Here's the drawing with two shaded views (mm, measured from the low corner). I have some questions. A direction names the side the tool comes from. Coordinates: 2 decimals unless noted, no trailing zeros. Order: outer loops, then holes, each group sorted by start corner. A loop starts at its lowest first (then second) coordinate and runs counter-clockwise, first axis right, second up. Notation, with made-up numbers: (-9.75, 59.25) -> (13.25, 59.25) arc R24 cw to (13.25, 83.25) -> close; hole circle Ø6 at (34, -13.75). An arc over 180 degrees is marked (long way). Return JSON: item names as keys, results as strings. Group by question number.
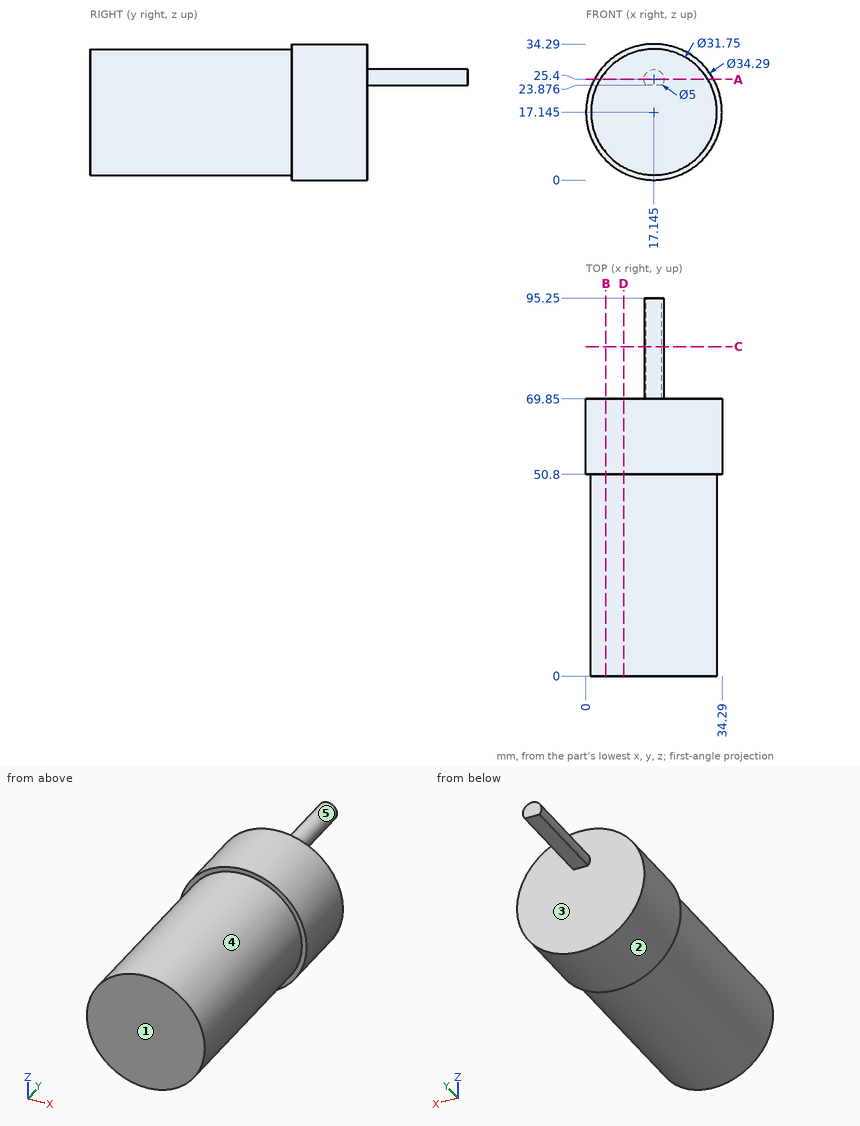
Q1. I want a section at C-C on y = 83. Please give me the cut outline in (x, z) (3 decimals), and give its area (3 significant figures).
Q2. We'd pull the mould along Y, two halves only. Please class the marked faces 1, 2 and 3: pulls with the +Y half, pulls with the -Y half, needs draft (parallel to the pull), parting line crosses it, or undercut.
Q3. I need wall thicknesses on line 1 along Z through (x, y) = (17.5, 6.5); line 2 along Y through (x, z) = (28.5, 27); line 3 along Y through (x, z) = (2, 24.5). Which ranges of each line are inside material? Lowest first, please. Write a range as from..to.
Q4. I want a section at A-A on z = 25.4. Please give me the cut outline in (x, y) (3 decimals), and give its area (3 significant figures).
Q5. I'm going to push flat-ended pins straight in: pin 1 Ø5 at (x, z) = (20.5, 7) entering from +Y; pin 2 Ø6 at (x, y) = (23.5, 37) entering from -Z; pin 3 Ø4 at (x, y) = (22.5, 61) entering from -Z. Where does each tip first touch, or does it pass through?
Q6. On a 3-axis mill with a long thin cutter (end or side, diameter ignored), from which of +Z, -Z, +X, -X, +Y, -Y can I reach the whole of each face in a straight line? I mean the marked faces 4 and 5. Say none if no direction works.
Q7. I want a section at D-D on x = 9.5. Please give me the cut outline in (y, z), and give its area (3 significant figures).
Q8. I want a section at B-B on x = 5. Please give me the cut outline in (y, z), and give its area (3 significant figures).
Response values:
{
 "1": {"outline": "(15.163, 23.876) -> (19.127, 23.876) arc R2.5 ccw (long way) to start", "area": "16.9 mm²"},
 "2": {"face 1": "pulls with the -Y half", "face 2": "needs draft", "face 3": "pulls with the +Y half"},
 "3": {"line 1": "z = 1.27..33.02", "line 2": "y = 0..69.85", "line 3": "y = 50.8..69.85"},
 "4": {"outline": "(2.118, 50.8) -> (3.585, 50.8) -> (3.585, 0) -> (30.705, 0) -> (30.705, 50.8) -> (32.172, 50.8) -> (32.172, 69.85) -> (19.645, 69.85) -> (19.645, 95.25) -> (14.645, 95.25) -> (14.645, 69.85) -> (2.118, 69.85) -> close", "area": "2,080 mm²"},
 "5": {"pin 1": "stops at y = 69.85", "pin 2": "stops at z = 1.63", "pin 3": "stops at z = 0.33"},
 "6": {"face 4": "-Y", "face 5": "+Y"},
 "7": {"outline": "(0, 3.23) -> (50.8, 3.23) -> (50.8, 1.8) -> (69.85, 1.8) -> (69.85, 32.49) -> (50.8, 32.49) -> (50.8, 31.06) -> (0, 31.06) -> close", "area": "2,000 mm²"},
 "8": {"outline": "(0, 6.92) -> (50.8, 6.92) -> (50.8, 5.04) -> (69.85, 5.04) -> (69.85, 29.25) -> (50.8, 29.25) -> (50.8, 27.37) -> (0, 27.37) -> close", "area": "1,500 mm²"}
}
